The listing builds one solid part. Answer for the finished solid, in the listing's coordinates (mm). Face numbers are marked on the shaded views. Coordinates: 2 decimals unless noted, no trailing zeros. Order: outer loops, then holes, each group sorted by start corner. A loop starts at its lowest first (then second) coordinate and runs counter-clockwise, first axis right, second up. Notation, with made-up numbers: (5.5, 68.5) - (63.5, 68.5) arc R31 ccw to (63.5, 104.5) - close; hole circle Ø10 at (20.25, 39). An arc over 180 degrees is marked (long way). One line per item, written item: value. Start each with the question number.
```python
from build123d import *

# Parameters (mm, degrees)
SKETCH_1_W          = 100
SKETCH_1_H          = 80
EXTRUDE_1_DEPTH     = 60
SKETCH_2_R          = 10
CUT_EXTRUDE_1_DEPTH = 3
SKETCH_3_R          = 6
CUT_EXTRUDE_2_DEPTH = 40
SKETCH_4_R          = 8
CUT_EXTRUDE_3_DEPTH = 8
SKETCH_5_R          = 5
CUT_EXTRUDE_4_DEPTH = 70
SKETCH_6_R          = 5
CUT_EXTRUDE_5_DEPTH = 40
SKETCH_7_R          = 7
CUT_EXTRUDE_6_DEPTH = 45
SKETCH_8_R          = 5
CUT_EXTRUDE_7_DEPTH = 30
SKETCH_9_R          = 4.5
CUT_EXTRUDE_8_DEPTH = 101
SKETCH_10_R         = 2.1
CUT_EXTRUDE_9_DEPTH = 10


with BuildPart() as part:
    # 草图1 → 凸台-拉伸1 (new body)
    with BuildSketch(Plane.XY):
        Rectangle(SKETCH_1_W, SKETCH_1_H)
    extrude(amount=EXTRUDE_1_DEPTH)

    # 草图2 → 切除-拉伸1 (cut)
    with BuildSketch(Plane.XY.offset(60)):
        with Locations((-25, 0)):
            Circle(SKETCH_2_R)
    extrude(amount=-CUT_EXTRUDE_1_DEPTH, mode=Mode.SUBTRACT)

    # 草图3 → 切除-拉伸2 (cut)
    with BuildSketch(Plane.XY.offset(60)):
        with Locations((-25, 0)):
            Circle(SKETCH_3_R)
    extrude(amount=-CUT_EXTRUDE_2_DEPTH, mode=Mode.SUBTRACT)

    # 草图4 → 切除-拉伸3 (cut)
    with BuildSketch(Plane(origin=(-50, 0, 0), x_dir=(0, 0, -1), z_dir=(1, 0, 0))):
        with Locations((-20, 0)):
            Circle(SKETCH_4_R)
    extrude(amount=CUT_EXTRUDE_3_DEPTH, mode=Mode.SUBTRACT)

    # 草图5 → 切除-拉伸4 (cut)
    with BuildSketch(Plane(origin=(-50, 0, 0), x_dir=(0, 0, -1), z_dir=(1, 0, 0))):
        with Locations((-20, 0)):
            Circle(SKETCH_5_R)
    extrude(amount=CUT_EXTRUDE_4_DEPTH, mode=Mode.SUBTRACT)

    # 草图6 → 切除-拉伸5 (cut)
    with BuildSketch(Plane(origin=(0, 40, 0), x_dir=(1, 0, 0), z_dir=(0, 1, 0))):
        with Locations(Location((10, -20, 0), (0, 0, 270))):
            Circle(SKETCH_6_R)
    extrude(amount=-CUT_EXTRUDE_5_DEPTH, mode=Mode.SUBTRACT)

    # 草图7 → 切除-拉伸6 (cut)
    with BuildSketch(Plane.XY):
        with Locations(Location((25, -15, 0), (0, 0, 180))):
            Circle(SKETCH_7_R)
    extrude(amount=CUT_EXTRUDE_6_DEPTH, mode=Mode.SUBTRACT)

    # 草图8 → 切除-拉伸7 (cut)
    with BuildSketch(Plane(origin=(50, 0, 0), x_dir=(0, 0, -1), z_dir=(1, 0, 0))):
        with Locations((-35, -15)):
            Circle(SKETCH_8_R)
    extrude(amount=-CUT_EXTRUDE_7_DEPTH, mode=Mode.SUBTRACT)

    # 草图9 → 切除-拉伸8 (cut, symmetric)
    with BuildSketch(Plane.XY):
        with Locations((40, 30)):
            Circle(SKETCH_9_R)
        with Locations((40, -30)):
            Circle(SKETCH_9_R)
        with Locations((-40, 30)):
            Circle(SKETCH_9_R)
        with Locations((-40, -30)):
            Circle(SKETCH_9_R)
    extrude(amount=CUT_EXTRUDE_8_DEPTH, both=True, mode=Mode.SUBTRACT)

    # 草图10 → 切除-拉伸9 (cut)
    with BuildSketch(Plane.XY.offset(60)):
        with Locations((-9, 16)):
            Circle(SKETCH_10_R)
        with Locations((-9, -16)):
            Circle(SKETCH_10_R)
        with Locations((-41, 16)):
            Circle(SKETCH_10_R)
        with Locations((-41, -16)):
            Circle(SKETCH_10_R)
    extrude(amount=-CUT_EXTRUDE_9_DEPTH, mode=Mode.SUBTRACT)


solid = part.part
```
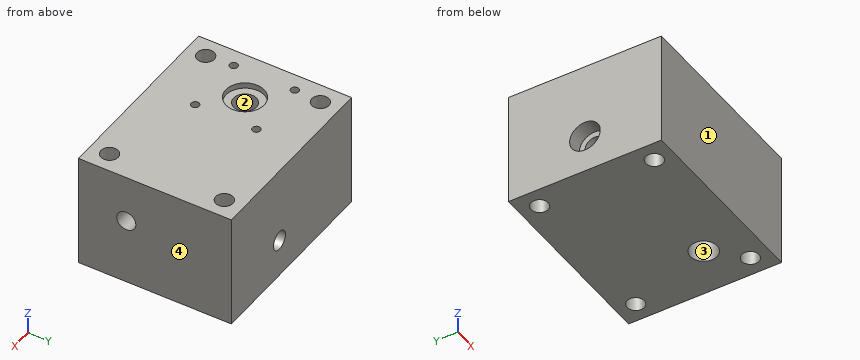
(1) The part is cut by section B-B on z = 10.5. Determine the outline of the cut face in (x, y).
(2) The part is cut by section C-C on x = 10. Determine the outline of the cut face in (y, z).
(3) Consider probe 1 along Y at (x, z) = (-40, 47); probe 2 along X at (y, z) = (30, 33); probe 3 along Y at (x, z) = (-9, 56.5). Determine where each line is inside the solid, lowest interval first.
(4) The part is cut by section D-D on z = 52.5. Count the separate pieces of the cut face and the enclosed holes in it, plus the area to 3 significant figures.
(5) Flat-ended cylindrical pins translate along their axes: pin 1 Ø16 at (x, y) = (-25.5, 1.5) entering from +Z; pin 2 Ø13 at (y, z) = (0, 20) entering from -X. Find the tip coordinate at first contact, or state that the pin passes through.
(6) The part is cut by section A-A on x = 40. Determine the outline of the cut face in (y, z), plus the area to 3 significant figures.
(7) For a pull along Y with two mould halves and no side action, classify the marked faces 1, 2, 3 and 4 as pulls with the +Y half, pulls with the -Y half, needs draft (parallel to the pull), parting line crosses it, or undercut.
Completed:
1. outline: (-50, -40) - (50, -40) - (50, 40) - (-50, 40) - close; hole circle Ø9 at (-40, -30); hole circle Ø9 at (-40, 30); hole circle Ø14 at (25, -15); hole circle Ø9 at (40, -30); hole circle Ø9 at (40, 30)
2. outline: (-40, 0) - (40, 0) - (40, 15) - (0, 15) arc R5 cw to (0, 25) - (40, 25) - (40, 60) - (-40, 60) - close
3. probe 1: y = -40 to -34.5, -25.5 to 25.5, 34.5 to 40
3. probe 2: x = -50 to -44.5, -35.5 to 35.5, 44.5 to 50
3. probe 3: y = -40 to -18.1, -13.9 to 13.9, 18.1 to 40
4. separate pieces: 1
4. enclosed holes: 9
4. area: 7,580 mm2
5. pin 1: stops at z = 57
5. pin 2: stops at x = -42
6. outline: (-40, 0) - (-34.5, 0) - (-34.5, 60) - (-40, 60) - close; (-25.5, 0) - (25.5, 0) - (25.5, 60) - (-25.5, 60) - close; (34.5, 0) - (40, 0) - (40, 60) - (34.5, 60) - close; hole circle Ø10 at (-15, 35)
6. area: 3,640 mm2
7. face 1: pulls with the -Y half
7. face 2: undercut
7. face 3: undercut
7. face 4: needs draft
